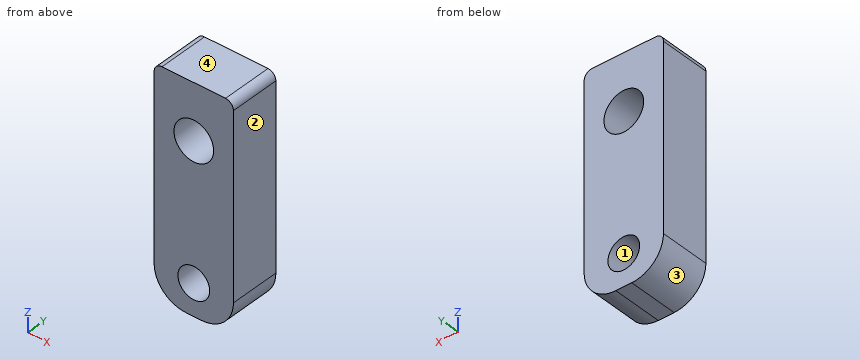
```python
from build123d import *

# Parameters (mm, degrees)
SKETCH2_W             = 5
SKETCH2_H             = 14
SKETCH2_R             = 1
BOSS_EXTRUDE1_DEPTH   = 3.175
M3X0_5_TAPPED_HOLE1_D = 2.5
FILLET1_R             = 2
FILLET2_R             = 0.5


with BuildPart() as part:
    # Sketch2 → Boss-Extrude1 (new body)
    with BuildSketch(Plane(origin=(0, 0, 0), x_dir=(1, 0, 0), z_dir=(0, 1, 0))):
        Rectangle(SKETCH2_W, SKETCH2_H)
        with Locations(Location((0, 5, 0), (0, 0, 90))):
            Circle(SKETCH2_R, mode=Mode.SUBTRACT)
    extrude(amount=-BOSS_EXTRUDE1_DEPTH)

    # M3x0.5 Tapped Hole1 (through all)
    with Locations(Plane(origin=(0, 0, 0), x_dir=(1, 0, 0), z_dir=(0, 1, 0))):
        with Locations((0, -3.5)):
            Hole(M3X0_5_TAPPED_HOLE1_D / 2)

    # Fillet1
    fillet1_edges = [part.edges().sort_by_distance(p)[0] for p in [
        (-2.5, -1.5875, -7),
        (2.5, -1.5875, -7),
    ]]
    fillet(fillet1_edges, radius=FILLET1_R)

    # Fillet2
    fillet2_edges = [part.edges().sort_by_distance(p)[0] for p in [
        (2.5, -1.5875, 7),
        (-2.5, -1.5875, 7),
    ]]
    fillet(fillet2_edges, radius=FILLET2_R)


solid = part.part
```
The model under review builds one solid part; all positions refer to its coordinate system, in mm. Face numbers are marked on the shaded views. Give positions to 0.01 mm unless a question says otherwise; leave off trailing zeros. Write each loop counter-clockwise with the first axis right and the second up, starting at its lowest first coordinate (ties: lowest second). Pieces come first, ordered by that corner, then holes. Notation, with made-up numbers: (57, -11) -> (88, -11) arc R21 ccw to (88, 23) -> close; hole circle Ø6 at (-2, 7.5). An arc over 180 degrees is marked (long way). Put each result on its own line as item: value.
(1) The part is to be moulded in two halves that separate along Z. For the marked faces 1, 2, 3 and 4, say which applies: pulls with the +Z half, pulls with the -Z half, needs draft (parallel to the pull), parting line crosses it, or undercut.
Results are:
face 1: undercut
face 2: needs draft
face 3: pulls with the -Z half
face 4: pulls with the +Z half
(2) We need section B-B, the plane y = -1.6. Give the boundary of the cut face in (x, z), and give its area (3 significant figures).
Results are:
outline: (-2.5, -5) arc R2 ccw to (-0.5, -7) -> (0.5, -7) arc R2 ccw to (2.5, -5) -> (2.5, 6.5) arc R0.5 ccw to (2, 7) -> (-2, 7) arc R0.5 ccw to (-2.5, 6.5) -> close; hole circle Ø2.5 at (0, 3.5); hole circle Ø2 at (0, -5)
area: 60.1 mm²
(3) We need section C-C, the plane z = 3.5. Give the boundary of the cut face in (x, y) (3 decimals).
Results are:
outline: (-2.5, -3.175) -> (-1.25, -3.175) -> (-1.25, 0) -> (-2.5, 0) -> close; (1.25, -3.175) -> (2.5, -3.175) -> (2.5, 0) -> (1.25, 0) -> close
(4) We need section A-A, the plane x = 0. Give the boundary of the cut face in (y, z) (3 decimals), and give its area (3 significant figures).
Results are:
outline: (-3.175, -7) -> (0, -7) -> (0, -6) -> (-3.175, -6) -> close; (-3.175, -4) -> (0, -4) -> (0, 2.25) -> (-3.175, 2.25) -> close; (-3.175, 4.75) -> (0, 4.75) -> (0, 7) -> (-3.175, 7) -> close
area: 30.2 mm²
(5) For pin 1 Ø1 at (x, y) = (1.5, -1.5) entering from -Z; pin 2 Ø3 at (x, z) = (0, 3.5) entering from -Y (3 decimals), all flat-tipped, find the tip position at first contact; note any pin that passes through.
Results are:
pin 1: z = -6.94
pin 2: y = -3.175
(6) To check wall thickness, follow probe 1 along Z at (x, y) = (0.05, -0.4); probe 2 along Z at (x, y) = (0.8, -1.3); probe 3 along X at (y, z) = (-0.25, 4.25). State the ranges of each line that lie inside material, in increasing order. Write a range as from..to.
Results are:
probe 1: -7..-6, -4..2.25, 4.75..7
probe 2: -6.98..-5.6, -4.4..2.54, 4.46..7
probe 3: -2.5..-1, 1..2.5
(7) We need section D-D, the plane x = -0.7. Give the boundary of the cut face in (y, z) (3 decimals).
Results are:
outline: (-3.175, -6.99) -> (0, -6.99) -> (0, -5.714) -> (-3.175, -5.714) -> close; (-3.175, -4.286) -> (0, -4.286) -> (0, 2.464) -> (-3.175, 2.464) -> close; (-3.175, 4.536) -> (0, 4.536) -> (0, 7) -> (-3.175, 7) -> close
